Geometry: final body of the model. Coordinates: model frame, mm. Round coordinates to 2 decimals unless told otherwise and drop trailing zeros. Loops run counter-clockwise (first coordinate to the right, second up) from the corner with the lowest first, then second, coordinate; pieces in that order, holes last. Notation, with made-up numbers: M -19,40.5 L -11,40.5 A33 cw -11,76.5 Z; hole C 85.25,11.5 d1. An arc over 180 degrees is marked long. Answer as a JSON object with one key per item and string values.
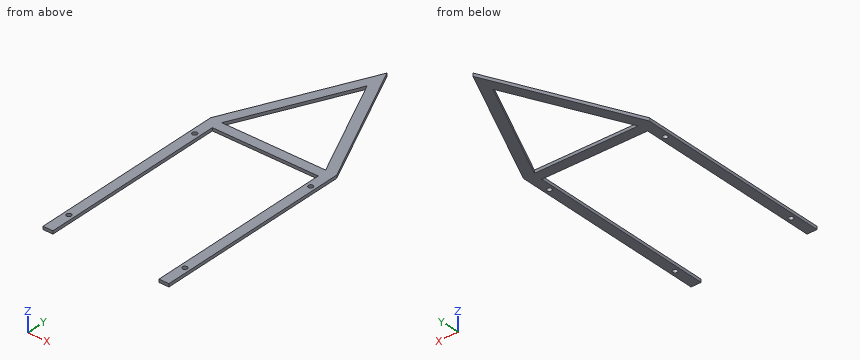
```python
from build123d import *

# Parameters (mm, degrees)
RECTANGLE_RIB_DEPTH                  = 1.5
TRIANGLE_RIB_DEPTH                   = 3
M4_CLEARANCE_HOLE1_D                 = 4.8
MIRROR1_AT_THE_SECOND_PLANE_COPY_1_D = 4.8


with BuildPart() as part:
    # Sketch1 → Rectangle Rib (new, symmetric)
    with BuildSketch(Plane.XY):
        Polygon((-63, -100), (-53, -100), (-53, -90), (-53, 90), (53, 90), (53, -90), (53, -100), (63, -100), (63, 100), (-63, 100), align=None)
    extrude(amount=RECTANGLE_RIB_DEPTH, both=True)

    # Sketch2 → Triangle Rib (add)
    with BuildSketch(Plane.XY.offset(1.5)):
        Polygon((-63, 100), (0, 235.103935992), (63, 100), (51.96622081, 100), (0, 211.441920161), (-51.96622081, 100), align=None)
    extrude(amount=-TRIANGLE_RIB_DEPTH)

    # M4 Clearance Hole1 (through all)
    with Locations(Plane.XY.offset(1.5)):
        with Locations((-58, 75)):
            m4_clearance_hole1 = Hole(M4_CLEARANCE_HOLE1_D / 2)

    # Mirror1: M4 Clearance Hole1 across plane
    add(m4_clearance_hole1.mirror(Plane.ZX), mode=Mode.SUBTRACT)

    # Mirror1 at the second plane: M4 Clearance Hole1 across plane
    add(m4_clearance_hole1.mirror(Plane(origin=(0, 0, 0), x_dir=(0, 0, 1), z_dir=(1, 0, 0))), mode=Mode.SUBTRACT)

    # Mirror1 at the second plane copy 1 (through all)
    with Locations(Plane(origin=(0, 0, 1.5), x_dir=(-1, 0, 0), z_dir=(0, 0, 1))):
        with Locations((-58, 75)):
            Hole(MIRROR1_AT_THE_SECOND_PLANE_COPY_1_D / 2)


solid = part.part
```
1) Cut plane B-B on z = -1.05. Return the cut outline in (x, y).
Geometry results:
{"outline": "M -63,-100 L -53,-100 L -53,90 L 53,90 L 53,-100 L 63,-100 L 63,100 L 0,235.1 L -63,100 Z; hole C -58,-75 d4.8; hole C -58,75 d4.8; hole M -51.97,100 L 51.97,100 L 0,211.44 Z; hole C 58,-75 d4.8; hole C 58,75 d4.8"}
2) Cut plane A-A on y = 62. Return the cut outline in (x, z), and give its area (3 significant figures).
Geometry results:
{"outline": "M -63,-1.5 L -53,-1.5 L -53,1.5 L -63,1.5 Z; M 53,-1.5 L 63,-1.5 L 63,1.5 L 53,1.5 Z", "area": "60.0 mm2"}
3) First-contact query: pin 1 (1.5 mm diameter, centred on x = -22, z = -0.5, fed in from -Y); pin 2 (1.5 mm diameter, centred on x = 16.5, z = 0.5, fed in from +Y). Flat tips, straight axial feed; report the tip coordinate or a pass-through.
Geometry results:
{"pin 1": "y = 90", "pin 2": "y = 201.33"}
4) Cut plane C-C on x = -34. Return the cut outline in (y, z), and give its area (3 significant figures).
Geometry results:
{"outline": "M 90,-1.5 L 100,-1.5 L 100,1.5 L 90,1.5 Z; M 138.53,-1.5 L 162.19,-1.5 L 162.19,1.5 L 138.53,1.5 Z", "area": "101 mm2"}
5) Line query: probe 1 along X at (y, z) = (-21, 1.3); probe 2 along Y at (x, z) = (58, 0.4); probe 3 along X at (y, z) = (162.5, 1.2). Output: solid intervals per line, ascending.
Geometry results:
{"probe 1": "-63 to -53, 53 to 63", "probe 2": "-100 to -77.4, -72.6 to 72.6, 77.4 to 110.72", "probe 3": "-33.86 to -22.82, 22.82 to 33.86"}
